For this review, take the finished solid that the model builds, in its own axes (mm). Round coordinates to 2 decimals unless told otherwise and drop trailing zeros. Write each loop counter-clockwise with the first axis right and the second up, starting at its lowest first coordinate (ties: lowest second). Pieces come first, ordered by that corner, then holes.
Autodesk Inventor part; units mm, degrees
ref_plane "YZ Plane" through (0, 0, 0) normal (1, 0, 0) x (0, 1, 0)
ref_plane "XZ Plane" through (0, 0, 0) normal (0, 1, 0) x (-1, 0, 0)
ref_plane "XY Plane" through (0, 0, 0) normal (0, 0, 1) x (1, 0, 0)
sketch "Sketch1" plane through (0, 0, 0) normal (0, 0, 1) x (1, 0, 0)
  line L0 (0, 0) -> (100, 0)
  line L1 (100, 0) -> (100, 95)
  line L2 (100, 95) -> (0, 95)
  line L3 (0, 95) -> (0, 0)
  point P0 (10, 10)
  point P1 (90, 10)
  point P2 (90, 85)
  point P3 (10, 85)
  dimension "d0" = 100
  dimension "d1" = 95
  dimension "d4" = 75
  dimension "d5" = 10
  dimension "d6" = 80
  dimension "d7" = 10
extrude "Extrusion1" add sketch "Sketch1" along normal blind 5
hole "Hole1" at (10, 10, 0) at (90, 10, 0) at (90, 85, 0) at (10, 85, 0) direction (0, 0, 1) diameter 6 end through all
sketch "Sketch2" plane through (0, 0, 0) normal (0, 0, -1) x (-1, 0, 0)
  line L0 (0, 95) -> (0, 0)
  line L1 (-100, 95) -> (0, 95)
  line L2 (-75, 33.401) -> (-75, 18.401) construction
  line L3 (-72, 33.401) -> (-72, 18.401)
  line L4 (-78, 18.401) -> (-78, 33.401)
  arc A0 (-72, 33.401) -> (-78, 33.401) centre (-75, 33.401) ccw
  arc A1 (-78, 18.401) -> (-72, 18.401) centre (-75, 18.401) ccw
  line L5 (-50, 33.401) -> (-50, 18.401) construction
  line L6 (-53, 33.401) -> (-53, 18.401)
  line L7 (-47, 18.401) -> (-47, 33.401)
  arc A2 (-47, 33.401) -> (-53, 33.401) centre (-50, 33.401) ccw
  arc A3 (-53, 18.401) -> (-47, 18.401) centre (-50, 18.401) ccw
  line L8 (-25, 33.401) -> (-25, 18.401) construction
  line L9 (-22, 33.401) -> (-22, 18.401)
  line L10 (-28, 18.401) -> (-28, 33.401)
  arc A4 (-22, 33.401) -> (-28, 33.401) centre (-25, 33.401) ccw
  arc A5 (-28, 18.401) -> (-22, 18.401) centre (-25, 18.401) ccw
  point P0 (-25, 25.901)
  point P1 (-50, 25.901)
  point P2 (-75, 25.901)
  point P3 (-75, 25.901)
  point P4 (-50, 25.901)
  point P5 (-25, 25.901)
  dimension "d15" = 50
  dimension "d17" = 25
  dimension "d18" = 25
  dimension "d19" = 69.099
  dimension "d27" = 6
  dimension "d28" = 15
  dimension "d29" = 7.5
extrude "Extrusion2" cut sketch "Sketch2" against normal blind 10
properties part number "Magazine_Mount_Plate_3DPrint"
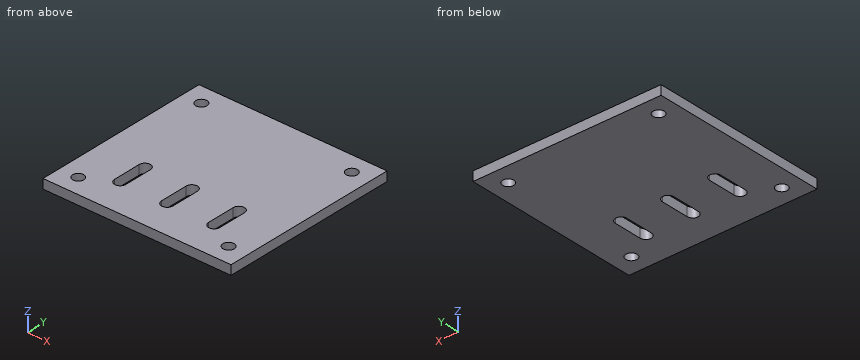
(1) For line 1 along Y through (x, z) = (10, 1.5); line 2 along X through (y, z) = (85, 3.95); line 3 along X through (y, z) = (26, 1.9), list the stretches that pass through material, from the lowest coordinate up.
Geometry check:
line 1: y = 0 to 7, 13 to 82, 88 to 95
line 2: x = 0 to 7, 13 to 87, 93 to 100
line 3: x = 0 to 22, 28 to 47, 53 to 72, 78 to 100
(2) We need section D-D, the plane y = 10. Give the boundary of the cut face in (x, z).
Geometry check:
outline: (0, 0) - (7, 0) - (7, 5) - (0, 5) - close; (13, 0) - (87, 0) - (87, 5) - (13, 5) - close; (93, 0) - (100, 0) - (100, 5) - (93, 5) - close
(3) We need section B-B, the plane y = 20. Give the boundary of the cut face in (x, z), and give its area (3 significant figures).
Geometry check:
outline: (0, 0) - (22, 0) - (22, 5) - (0, 5) - close; (28, 0) - (47, 0) - (47, 5) - (28, 5) - close; (53, 0) - (72, 0) - (72, 5) - (53, 5) - close; (78, 0) - (100, 0) - (100, 5) - (78, 5) - close
area: 410 mm2
(4) We need section A-A, the plane x = 90. Give the boundary of the cut face in (y, z).
Geometry check:
outline: (0, 0) - (7, 0) - (7, 5) - (0, 5) - close; (13, 0) - (82, 0) - (82, 5) - (13, 5) - close; (88, 0) - (95, 0) - (95, 5) - (88, 5) - close
(5) We need section C-C, the plane x = 75. Give the boundary of the cut face in (y, z), and give its area (3 significant figures).
Geometry check:
outline: (0, 0) - (15.4, 0) - (15.4, 5) - (0, 5) - close; (36.4, 0) - (95, 0) - (95, 5) - (36.4, 5) - close
area: 370 mm2
(6) For pin 1 Ø5.5 at (x, y) = (90, 10) entering from +Z; pin 2 Ø2.5 at (y, z) = (26, 2.5) entering from -X, all flat-tipped, find the tip position at first contact; note any pin that passes through.
Geometry check:
pin 1: passes through
pin 2: stops at x = 0
